Build history of the part. All positions in model axes, mm. Face numbers are marked on the shaded views. A direction names the side the tool comes from. Coordinates: 2 decimals unless noted, no trailing zeros. Loops run counter-clockwise (first coordinate to the right, second up) from the corner with the lowest first, then second, coordinate; pieces in that order, holes last.
(1) Slice it at D-D (y = 25). Give the cut face in (x, z).
(2) Wall check: L1, parallel to X at y = 2.5, z = 5.08; L2, parallel to Z at x = 20, y = 27; L3, parallel to X at y = 5, z = -20. Give the ranges that are in metal, low to high.
(3) Two-plate mould, pull along X, no slides. Class the marked faces 1, 2 and 3: pulls with the +X half, pulls with the -X half, needs draft (parallel to the pull), parting line crosses it, or undercut.
(4) Slice it at B-B (z = -20.32). Give the cut face in (x, y).
(5) Flat gauge pins, fed straight in: P1, Ø5, axis at x = -0.5, y = 18.5, coming from the -Z side; P2, Ø6, axis at x = 15, y = 4, coming from the +Z side; P3, Ø3, axis at x = -5, z = -22, coming from the +Y side; P4, Ø1.9, axis at x = 47.5, y = 3, coming from the +Z side. Where does each tip first touch, or does it go through?
(6) Slice it at C-C (x = 20.32). Give the cut face in (y, z), and give its area (3 significant figures).
(7) Tool access for the marked faces 4, 5, 6, 7 and 8: list every direction of +Z, -Z, +X, -X, +Y, -Y with a clear straight run to the whole face (end or side of a thin tool).
(8) Slice it at A-A (x = -5.08). Give the cut face in (y, z), and give its area (3 significant figures).
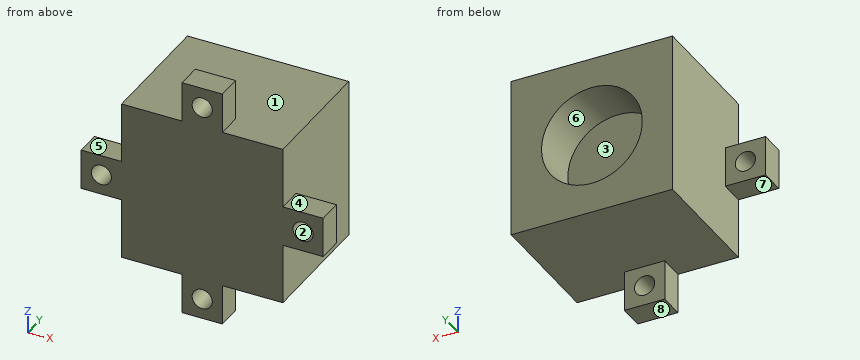
from build123d import *

# Parameters (mm, degrees)
SKETCH1_W           = 10.16
SKETCH1_H           = 10.16
SKETCH1_W_2         = 40.64
SKETCH1_H_2         = 40.64
BOSS_EXTRUDE1_DEPTH = 6.35
SKETCH2_R           = 2.54
CUT_EXTRUDE1_DEPTH  = 8.89
SKETCH3_W           = 40.64
SKETCH3_H           = 40.64
BODY_EXTRUDE_DEPTH  = 25.4
SKETCH4_R           = 12.7
MOTOR_HOLE_DEPTH    = 12.7


with BuildPart() as part:
    # Sketch1 → Boss-Extrude1 (new body)
    with BuildSketch(Plane(origin=(0, 0, 0), x_dir=(1, 0, 0), z_dir=(0, 1, 0))):
        with Locations((-5.08, 20.32)):
            Rectangle(SKETCH1_W, SKETCH1_H)
        with Locations((20.32, 45.72)):
            Rectangle(SKETCH1_W, SKETCH1_H)
        with Locations((20.32, 20.32)):
            Rectangle(SKETCH1_W_2, SKETCH1_H_2)
        with Locations((45.72, 20.32)):
            Rectangle(SKETCH1_W, SKETCH1_H)
        with Locations((20.32, -5.08)):
            Rectangle(SKETCH1_W, SKETCH1_H)
    extrude(amount=BOSS_EXTRUDE1_DEPTH)

    # Sketch2 → Cut-Extrude1 (cut)
    with BuildSketch(Plane(origin=(0, 6.35, 0), x_dir=(1, 0, 0), z_dir=(0, 1, 0))):
        with Locations((-5.08, 20.32)):
            Circle(SKETCH2_R)
        with Locations((20.32, 45.72)):
            Circle(SKETCH2_R)
        with Locations((45.72, 20.32)):
            Circle(SKETCH2_R)
        with Locations((20.32, -5.08)):
            Circle(SKETCH2_R)
    extrude(amount=-CUT_EXTRUDE1_DEPTH, mode=Mode.SUBTRACT)

    # Sketch3 → body_extrude (add)
    with BuildSketch(Plane(origin=(0, 6.35, 0), x_dir=(1, 0, 0), z_dir=(0, 1, 0))):
        with Locations((20.32, 20.32)):
            Rectangle(SKETCH3_W, SKETCH3_H)
    extrude(amount=BODY_EXTRUDE_DEPTH)

    # Sketch4 → motor_hole (cut)
    with BuildSketch(Plane(origin=(0, 31.75, 0), x_dir=(1, 0, 0), z_dir=(0, 1, 0))):
        with Locations((20.32, 20.32)):
            Circle(SKETCH4_R)
    extrude(amount=-MOTOR_HOLE_DEPTH, mode=Mode.SUBTRACT)


solid = part.part
Response values:
1. outline: (0, -40.64) - (40.64, -40.64) - (40.64, 0) - (0, 0) - close; hole circle Ø25.4 at (20.32, -20.32)
2. L1: x = 15.24 to 17.78, 22.86 to 25.4
2. L2: z = -40.64 to -33.02, -7.62 to 0
2. L3: x = -10.16 to -7.6, -2.56 to 43.2, 48.24 to 50.8
3. face 1: needs draft
3. face 2: undercut
3. face 3: undercut
4. outline: (-10.16, 0) - (-7.62, 0) - (-7.62, 6.35) - (-10.16, 6.35) - close; (-2.54, 0) - (43.18, 0) - (43.18, 6.35) - (40.64, 6.35) - (40.64, 31.75) - (33.02, 31.75) - (33.02, 19.05) - (7.62, 19.05) - (7.62, 31.75) - (0, 31.75) - (0, 6.35) - (-2.54, 6.35) - close; (48.26, 0) - (50.8, 0) - (50.8, 6.35) - (48.26, 6.35) - close
5. P1: stops at z = -40.64
5. P2: stops at z = 10.16
5. P3: stops at y = 6.35
5. P4: stops at z = -15.24
6. outline: (0, -50.8) - (6.35, -50.8) - (6.35, -48.26) - (0, -48.26) - close; (0, -43.18) - (6.35, -43.18) - (6.35, -40.64) - (31.75, -40.64) - (31.75, -33.02) - (19.05, -33.02) - (19.05, -7.62) - (31.75, -7.62) - (31.75, 0) - (6.35, 0) - (6.35, 2.54) - (0, 2.54) - close; (0, 7.62) - (6.35, 7.62) - (6.35, 10.16) - (0, 10.16) - close
6. area: 1,030 mm2
7. face 4: +Z, +X, +Y, -Y
7. face 5: +Z, -X, +Y, -Y
7. face 6: +Y
7. face 7: -Z, -X, +Y, -Y
7. face 8: -Z, +X, -X, +Y, -Y
8. outline: (0, -25.4) - (6.35, -25.4) - (6.35, -22.86) - (0, -22.86) - close; (0, -17.78) - (6.35, -17.78) - (6.35, -15.24) - (0, -15.24) - close
8. area: 32.3 mm2
